Input: part model. Units: mm. Frame: model coordinates. A direction names the side the tool comes from. Give positions to 0.01 mm unless a question says otherwise; leave off trailing zeros. Loops run counter-clockwise (first coordinate to the right, second up) from the corner with the lowest first, then second, coordinate; pieces in that order, holes last. Notation, with made-up numbers: (49.25, 26) -> (68.25, 26) arc R10 cw to (68.25, 32) -> close; hole circle Ø3 at (2, -36). An arc over 180 degrees is marked (long way). Answer as a JSON object with one key per item and string values. Group by question number.
Solid Edge part; units mm, degrees
sketch "Sketch1" plane through (0, 0, 0) normal (0, 0, 1) x (1, 0, 0)
  line L0 (-10.5, 51) -> (-10.5, -18)
  arc A0 (10.5, -18) -> (-10.5, -18) centre (0, -18) cw
  line L1 (10.5, -18) -> (10.5, 51)
  arc A1 (-10.5, 51) -> (10.5, 51) centre (0, 51) cw
  dimension "D1" = 10.5
extrude "Protrusion1" add sketch "Sketch1" along normal mid plane 8
sketch "Sketch2" plane through (0, 39.5, -4) normal (0, 0, -1) x (0, -1, 0)
  circle A0 centre (57.5, 0) radius 1.65
  circle A1 centre (-11.5, 0) radius 1.65
extrude "Cutout1" cut sketch "Sketch2" against normal up to next
sketch "Sketch3" plane through (0, -5.25, 4) normal (0, 0, 1) x (0, 1, 0)
  circle A0 centre (56.25, 0) radius 2.875
  circle A1 centre (-12.75, 0) radius 2.875
extrude "VaciadoExtruido_4" cut sketch "Sketch3" against normal blind 3
sketch "Sketch4" plane through (10.5, 16.5, 0) normal (1, 0, 0) x (0, 1, 0)
  circle A0 centre (-20.5, 0) radius 1.65
  circle A1 centre (-12.5, 0) radius 1.65
extrude "Cutout2" cut sketch "Sketch4" against normal through all
fillet "Redondeo_2" radius 2 4 edges at (0, -28.5, 4) (10.5, 16.5, 4) (0, 61.5, 4) (-10.5, 16.5, 4)
sketch "Sketch5" plane through (10.5, 16.5, -1) normal (1, 0, 0) x (0, -1, 0)
  line L0 (18.9123, 1.75) -> (22.0877, 1.75)
  line L1 (22.0877, 1.75) -> (23.6754, -1)
  line L2 (23.6754, -1) -> (22.0877, -3.75)
  line L3 (22.0877, -3.75) -> (18.9123, -3.75)
  line L4 (18.9123, -3.75) -> (17.3246, -1)
  line L5 (17.3246, -1) -> (18.9123, 1.75)
  line L6 (10.9123, 1.75) -> (14.0877, 1.75)
  line L7 (14.0877, 1.75) -> (15.6754, -1)
  line L8 (15.6754, -1) -> (14.0877, -3.75)
  line L9 (14.0877, -3.75) -> (10.9123, -3.75)
  line L10 (10.9123, -3.75) -> (9.3246, -1)
  line L11 (9.3246, -1) -> (10.9123, 1.75)
extrude "VaciadoExtruido_23" cut sketch "Sketch5" against normal blind 3
properties material "Abs 15"
Q1. Section A-A on x = 0. Return the cut outline in (y, z) (3 decimals), then the cut area to 3 significant figures.
Q2. Ray query, probe 1 along Y at (x, z) = (0, -0.25); probe 2 along Y at (x, z) = (1.5, 2.25); probe 3 along Y at (x, z) = (-3.5, 1). Return the intervals inside material, ascending.
Q3. Section B-B on y = 4. Return the cut outline in (x, z).
Q4. Pin query (flat end, axial travel): pin 1 Ø4.5 at (y, z) = (-4, 0) entering from +X; pin 2 Ø2 at (y, z) = (4, 0) entering from +X; pin 3 Ø2 at (x, z) = (-5.5, -1.5) entering from -Y. Return the tip coordinate at first contact, or that it passes through.
Q5. Set-up query: faces 4 (the face through (-0.126, 48.128, 2.521)), 5 (the face through (9.02, 6.39, -1.36)), 6 (the face through (10.5, 16, -1)). Return all of +Z, -Z, +X, -X, +Y, -Y with unobstructed straight access to the full face (end or side cutting, diameter ignored); none if empty.
Q6. Pull-direction query (Y, two-part tool) for faces 1 (the face through (-0.2, 61.5, -1)), 2 (the face through (-9.93, 16.98, 3.4)), 3 (the face through (-1.37, -5.65, 0.07)); classes: +Y half, -Y half, draft (parallel to the pull), parting line (faces both ways), or undercut.
Numbers:
{
 "1": {"outline": "(-28.5, -4) -> (-19.65, -4) -> (-19.65, 1) -> (-20.875, 1) -> (-20.875, 4) -> (-26.5, 4) arc R2 ccw to (-28.5, 2) -> close; (-16.35, -4) -> (49.35, -4) -> (49.35, 1) -> (48.125, 1) -> (48.125, 4) -> (-15.125, 4) -> (-15.125, 1) -> (-16.35, 1) -> close; (52.65, -4) -> (61.5, -4) -> (61.5, 2) arc R2 ccw to (59.5, 4) -> (53.875, 4) -> (53.875, 1) -> (52.65, 1) -> close; hole circle Ø3.3 at (-4, 0); hole circle Ø3.3 at (4, 0)", "area": "634 mm²"},
 "2": {"probe 1": "y = -28.5 to -19.65, -16.35 to -5.63, -2.37 to 2.37, 5.63 to 49.35, 52.65 to 61.5", "probe 2": "y = -28.38 to -20.45, -15.55 to 48.55, 53.45 to 61.38", "probe 3": "y = -27.9 to -5.31, -2.69 to 2.69, 5.31 to 60.9"},
 "3": {"outline": "(-10.5, -4) -> (10.5, -4) -> (10.5, -2.75) -> (7.5, -2.75) -> (7.5, -1.65) -> (-10.5, -1.65) -> close; (-10.5, 1.65) -> (7.5, 1.65) -> (7.5, 2.75) -> (10.35, 2.75) arc R2 ccw to (8.5, 4) -> (-8.5, 4) arc R2 ccw to (-10.5, 2) -> close"},
 "4": {"pin 1": "stops at x = 7.5", "pin 2": "passes through", "pin 3": "stops at y = -27.49"},
 "5": {"face 4": "+Z", "face 5": "+X", "face 6": "+Z, -Z, +X, +Y, -Y"},
 "6": {"face 1": "+Y half", "face 2": "draft", "face 3": "undercut"}
}
